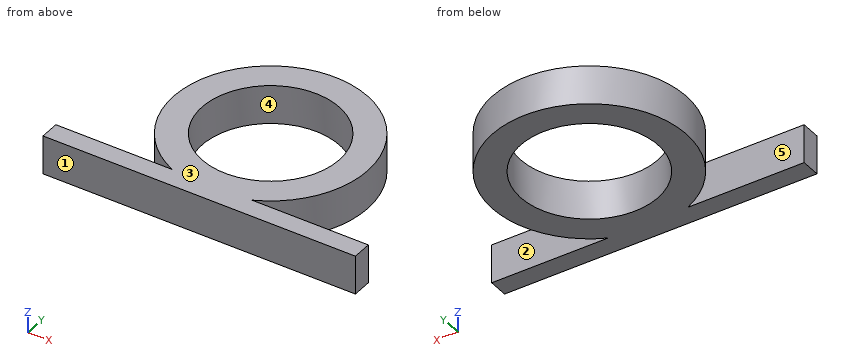
Autodesk Inventor part; units mm, degrees
ref_plane "YZ Plane" through (0, 0, 0) normal (1, 0, 0) x (0, 1, 0)
ref_plane "XZ Plane" through (0, 0, 0) normal (0, 1, 0) x (-1, 0, 0)
ref_plane "XY Plane" through (0, 0, 0) normal (0, 0, 1) x (1, 0, 0)
sketch "スケッチ1" plane through (0, 0, 0) normal (0, 0, 1) x (1, 0, 0)
  circle A0 centre (0, 0) radius 17.7
  arc A1 (10.2674, -22.7943) -> (-10.2674, -22.7943) centre (0, 0) ccw
  line L0 (-10.2674, -22.7943) -> (-40.2674, -22.7943)
  line L1 (-40.2674, -22.7943) -> (-40.2674, -27.7943)
  line L2 (10.2674, -22.7943) -> (40.2674, -22.7943)
  line L3 (40.2674, -22.7943) -> (40.2674, -27.7943)
  line L4 (40.2674, -27.7943) -> (-40.2674, -27.7943)
  dimension "d0" = 35.4
  dimension "d1" = 25
  dimension "d2" = 30
  dimension "d3" = 5
  dimension "d4" = 30
  dimension "d5" = 5
extrude "押し出し1" add sketch "スケッチ1" along normal blind 10
properties part number "d35_hole"
Can you work these out from the model? Positions are in its coordinate system, mm. Face numbers are marked on the shaded views. A direction names the side the tool comes from. Give positions to 0.01 mm unless a question says otherwise; leave off trailing zeros. Write each loop counter-clockwise with the first axis right and the second up, starting at its lowest first coordinate (ties: lowest second). Pieces come first, ordered by that corner, then holes. Notation, with made-up numbers: M 53.25,16 L 70.25,16 A22 ccw 70.25,28 Z; hole C 18.25,59.5 d5. An arc over 180 degrees is marked long. Answer in a Markdown table with one row per item. Add a question column.
Item 1: Imagine slicing it at A-A, the plane x = 0. Write out the boundary of the cut face in (y, z), plus the area to 3 significant figures.
Item 2: Please list where these lines run through material, in increasing order: L1, parallel to Y at x = 15, z = 2; L2, parallel to Y at x = -28, z = 7; L3, parallel to X at y = -1, z = 7.5.
Item 3: For pin 1 Ø3 at (x, z) = (-32.5, 3) entering from +Y; pin 2 Ø5 at (x, z) = (16.5, 6.5) entering from +Y; pin 3 Ø2 at (y, z) = (16, 1.5) entering from +X, each with a flat end and sliding along its axis, tell me the tip position at first contact or that it passes through.
Item 4: Imagine slicing it at C-C, the plane z = 2. Write out the boundary of the cut face in (x, y).
Item 5: Imagine slicing it at D-D, the plane x = -28. Write out the boundary of the cut face in (y, z), plus the area to 3 significant figures.
Item 6: On a 3-axis mill with a long thin cutter (end or side, diameter ignored), from which of +Z, -Z, +X, -X, +Y, -Y can I reach the whole of each face in a straight line? I mean the marked faces 4 and 5. Say none if no direction works.
Item 7: Imagine slicing it at B-B, the plane y = 0. Write out the boundary of the cut face in (x, z), plus the area to 3 significant figures.
Item 8: We'd pull the mould along Y, two halves only. Please class the marked faces 1, 2 and 3: released by +Y, released by -Y, zero draft, split by the parting line, or undercut.
Evaluation:
| question | item | result |
|---|---|---|
| 1 | outline | M -27.79,0 L -17.7,0 L -17.7,10 L -27.79,10 Z; M 17.7,0 L 25,0 L 25,10 L 17.7,10 Z |
| 1 | area | 174 mm² |
| 2 | L1 | y = -27.79 to -22.79, -20 to -9.4, 9.4 to 20 |
| 2 | L2 | y = -27.79 to -22.79 |
| 2 | L3 | x = -24.98 to -17.67, 17.67 to 24.98 |
| 3 | pin 1 | stops at y = -22.79 |
| 3 | pin 2 | stops at y = 20.71 |
| 3 | pin 3 | stops at x = 20 |
| 4 | outline | M -40.27,-27.79 L 40.27,-27.79 L 40.27,-22.79 L 10.27,-22.79 A25 ccw long -10.27,-22.79 L -40.27,-22.79 Z; hole C 0,0 d35.4 |
| 5 | outline | M -27.79,0 L -22.79,0 L -22.79,10 L -27.79,10 Z |
| 5 | area | 50.0 mm² |
| 6 | face 4 | +Z, -Z |
| 6 | face 5 | +Z, -Z, -X |
| 7 | outline | M -25,0 L -17.7,0 L -17.7,10 L -25,10 Z; M 17.7,0 L 25,0 L 25,10 L 17.7,10 Z |
| 7 | area | 146 mm² |
| 8 | face 1 | released by -Y |
| 8 | face 2 | undercut |
| 8 | face 3 | zero draft |
